from build123d import *

# Parameters (mm, degrees)
SKETCH1_W           = 100
SKETCH1_H           = 104
BOSS_EXTRUDE1_DEPTH = 2
SKETCH2_R           = 1.5
CUT_EXTRUDE1_DEPTH  = 2
SKETCH3_W           = 28.414936843
SKETCH3_H           = 62.425741265
BOSS_EXTRUDE2_DEPTH = 40


with BuildPart() as part:
    # Sketch1 → Boss-Extrude1 (new body)
    with BuildSketch(Plane.XY):
        Rectangle(SKETCH1_W, SKETCH1_H)
    extrude(amount=BOSS_EXTRUDE1_DEPTH)

    # Sketch2 → Cut-Extrude1 (cut)
    with BuildSketch(Plane.XY.offset(2)):
        with Locations((-44, -37)):
            Circle(SKETCH2_R)
        with Locations((37, -37)):
            Circle(SKETCH2_R)
        with Locations((37, 39)):
            Circle(SKETCH2_R)
    extrude(amount=-CUT_EXTRUDE1_DEPTH, mode=Mode.SUBTRACT)

    # Sketch3 → Boss-Extrude2 (add)
    with BuildSketch(Plane.XY.offset(2)):
        with Locations((-31.124449574, 15.550972076)):
            Rectangle(SKETCH3_W, SKETCH3_H)
    extrude(amount=BOSS_EXTRUDE2_DEPTH)


solid = part.part
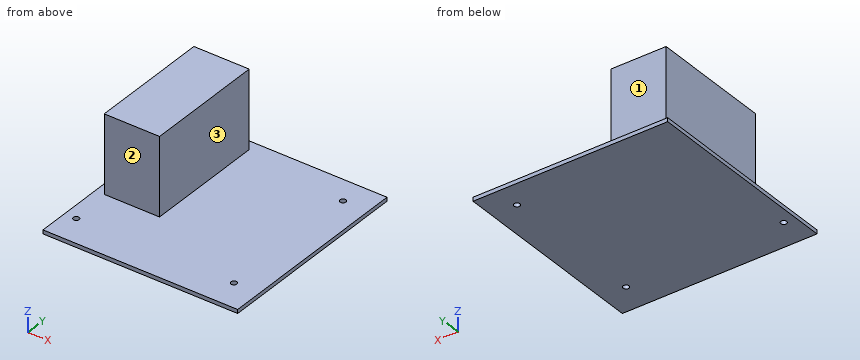
Verification items for the finished model (mm, model axes). Face numbers are marked on the shaded views. A direction names the side the tool comes from. Coordinates: 2 decimals unless noted, no trailing zeros. Order: outer loops, then holes, each group sorted by start corner. A loop starts at its lowest first (then second) coordinate and runs counter-clockwise, first axis right, second up. Notation, with made-up numbers: (24, -26) -> (37, -26) arc R27 ccw to (37, 10) -> close; hole circle Ø10 at (58, 74). An arc over 180 degrees is marked (long way). Put each result on its own line as item: value. Start each with the question number.
1. Material ranges on L1, parallel to Y at x = 37, z = 0.45; L2, parallel to Y at x = -31, z = 32; L3, parallel to Z at x = 22.5, y = -44.5, recorded low to high. Write a range as [from, to].
2. Cross-section at B-B, the plane x = -44. Record the boundary of the cut face in (y, z), then the cut area to 3 significant figures.
3. Go/stop test with flat-tipped pins: pin 1 Ø14 at (x, z) = (-37, 27) entering from +Y; pin 2 Ø1.8 at (x, y) = (37, 39) entering from -Z; pin 3 Ø2 at (y, z) = (1, 24) entering from +X; pin 4 Ø14 at (x, z) = (-27, 27) entering from -Y. Record where each tip stops, or that it passes through.
4. Cross-section at D-D, the plane y = 6.5. Record the boundary of the cut face in (x, z).
5. Access from +Z, -Z, +X, -X, +Y, -Y to the whole of each face (thin tool, end or side, straight path). Record for the marked faces 1, 2 and 3.
6. Cross-section at A-A, the plane y = -37. Record the boundary of the cut face in (x, z).
7. Cross-section at C-C, the plane y = 39. Record the boundary of the cut face in (x, z).
Computed:
1. L1: [-52, -38.5], [-35.5, 37.5], [40.5, 52]
1. L2: [-15.66, 46.76]
1. L3: [0, 2]
2. outline: (-52, 0) -> (-38.5, 0) -> (-38.5, 2) -> (-52, 2) -> close; (-35.5, 0) -> (52, 0) -> (52, 2) -> (46.76, 2) -> (46.76, 42) -> (-15.66, 42) -> (-15.66, 2) -> (-35.5, 2) -> close
2. area: 2,700 mm2
3. pin 1: y = 46.76
3. pin 2: through
3. pin 3: x = -16.92
3. pin 4: y = -15.66
4. outline: (-50, 0) -> (50, 0) -> (50, 2) -> (-16.92, 2) -> (-16.92, 42) -> (-45.33, 42) -> (-45.33, 2) -> (-50, 2) -> close
5. face 1: +Z, +X, -X, +Y
5. face 2: +Z, +X, -X, -Y
5. face 3: +Z, +X, +Y, -Y
6. outline: (-50, 0) -> (-45.5, 0) -> (-45.5, 2) -> (-50, 2) -> close; (-42.5, 0) -> (35.5, 0) -> (35.5, 2) -> (-42.5, 2) -> close; (38.5, 0) -> (50, 0) -> (50, 2) -> (38.5, 2) -> close
7. outline: (-50, 0) -> (35.5, 0) -> (35.5, 2) -> (-16.92, 2) -> (-16.92, 42) -> (-45.33, 42) -> (-45.33, 2) -> (-50, 2) -> close; (38.5, 0) -> (50, 0) -> (50, 2) -> (38.5, 2) -> close
